Autodesk Inventor part; units mm, degrees
ref_plane "YZ Plane" through (0, 0, 0) normal (1, 0, 0) x (0, 1, 0)
ref_plane "XZ Plane" through (0, 0, 0) normal (0, 1, 0) x (-1, 0, 0)
ref_plane "XY Plane" through (0, 0, 0) normal (0, 0, 1) x (1, 0, 0)
sketch "Sketch1" plane through (0, 0, 0) normal (0, 0, 1) x (1, 0, 0)
  line L0 (-2.6473, 22.1) -> (2.6473, 22.1)
  line L1 (2.6473, 22.1) -> (2.6473, 12)
  line L2 (2.6473, 12) -> (4.1473, 12)
  line L3 (4.1473, 12) -> (4.1473, 4.1473)
  line L4 (0, 22.1) -> (0, 0) construction
  line L5 (-2.6473, 22.1) -> (-2.6473, 12)
  line L6 (-2.6473, 12) -> (-4.1473, 12)
  line L7 (-1.25, 18.6) -> (1.25, 18.6)
  line L8 (1.25, 18.6) -> (1.25, 17.5)
  line L9 (1.25, 17.5) -> (-1.25, 17.5)
  line L10 (-1.25, 17.5) -> (-1.25, 18.6)
  line L11 (-9.6473, -24) -> (16.1473, -24)
  line L12 (26.1473, -9) -> (16.1473, -9)
  line L13 (16.1473, -9) -> (16.1473, -24)
  line L14 (3.0473, 2.1473) -> (4.1473, 2.1473)
  line L15 (4.1473, 2.1473) -> (4.1473, -0.3527)
  line L16 (4.1473, -0.3527) -> (3.0473, -0.3527)
  line L17 (3.0473, -0.3527) -> (3.0473, 2.1473)
  line L18 (-4.1473, 12) -> (-30.8527, 12) construction
  line L19 (-27.6, 2.6473) -> (-27.6, -2.6473)
  line L20 (-27.6, -2.6473) -> (-17.5, -2.6473)
  line L21 (-17.5, -2.6473) -> (-17.5, -4.1473)
  line L22 (-17.5, -4.1473) -> (-9.6473, -4.1473)
  line L23 (-9.6473, -4.1473) -> (-9.6473, -24)
  line L24 (-27.6, 2.6473) -> (-17.5, 2.6473)
  line L25 (-17.5, 2.6473) -> (-17.5, 4.1473)
  line L26 (-24.1, 1.25) -> (-24.1, -1.25)
  line L27 (-24.1, -1.25) -> (-23, -1.25)
  line L28 (-23, -1.25) -> (-23, 1.25)
  line L29 (-23, 1.25) -> (-24.1, 1.25)
  line L30 (-17.5, 12) -> (-17.5, -24) construction
  line L31 (-4.1473, 12) -> (-4.1473, 4.1473)
  line L32 (-9.6473, 4.1473) -> (-17.5, 4.1473)
  line L33 (-4.1473, 4.1473) -> (-9.6473, 4.1473)
  line L34 (26.1473, 4.1473) -> (26.1473, -9)
  line L35 (26.1473, -2.4263) -> (4.1473, -2.4263) construction
  line L36 (3.0473, -7) -> (4.1473, -7)
  line L37 (4.1473, -7) -> (4.1473, -4.5)
  line L38 (4.1473, -4.5) -> (3.0473, -4.5)
  line L39 (3.0473, -4.5) -> (3.0473, -7)
  line L40 (4.1473, 4.1473) -> (26.1473, 4.1473)
  point P0 (0, 17.5)
  point P1 (3.0473, 0.8973)
  point P2 (4.1473, 0.8973)
  point P3 (-24.1, 0)
  point P4 (-27.6, 0)
  dimension "d4" = 1.5
  dimension "d26" = 10.1
  dimension "d27" = 5.2946
  dimension "d31" = 2.5
  dimension "d32" = 1.1
  dimension "d35" = 5.5
  dimension "d41" = 1.1
  dimension "d42" = 2.5
  dimension "d72" = 17.5
  dimension "BearingHolderHeight" = 24.5263
  dimension "d99" = 5.5
  dimension "d103" = 12
  dimension "d104" = 10
  dimension "d105" = 13.1473
  dimension "d106" = 2
  dimension "d108" = 15
  dimension "d124" = 12
  dimension "d125" = 7.8527
extrude "Extrusion2" add sketch "Sketch1" along normal blind 6.39
equation "\"BearingDiameter\" = 24"
equation "\"WoodThickness\" = 6.39"
equation "\"BearingWidth\" = 7"
equation "\"BearingShaftDiameter\" = 8"
equation "\"ZipTieWidth\" = 2.5"
equation "\"ZipTieThickness\" = 1.1"
equation "\"ZipTieClearance\" = 1"
equation "\"ZipTieDistance\" = 10"
equation "\"BearingSiliconeWidth\" = 14"
properties part number "BearingStand_V2" material "Wood (Birch)"
Check sheet for the modelled part. Datum: model origin and axes. Units: mm. A direction names the side the tool comes from. Give positions to 0.01 mm unless a question says otherwise; leave off trailing zeros. Order: outer loops, then holes, each group sorted by start corner. A loop starts at its lowest first (then second) coordinate and runs counter-clockwise, first axis right, second up. Notation, with made-up numbers: M 36.25,-13.75 L 89.25,-13.75 A17 cw 89.25,15.25 Z; hole C -19,3 d10. An arc over 180 degrees is marked long. Answer in a Markdown table with one row per item.
1) Cross-section at B-B, the plane x = 19.5. Enter the section's corners in (y, z), plus the area to 3 significant figures.
Filled sheet:
| item | result |
|---|---|
| outline | M -9,0 L 4.15,0 L 4.15,6.39 L -9,6.39 Z |
| area | 84.0 mm2 |
2) Access from +Z, -Z, +X, -X, +Y, -Y to the whole of each face (thin tool, end or side, straight path). Record for faces 5 (the flat face through (15, 4.147, 3)), 6 (the flat face through (21, -9, 3)), 7 (the flat face through (-23.6, -1.25, 3.2)).
Filled sheet:
| item | result |
|---|---|
| face 5 | +Z, -Z, +X, +Y |
| face 6 | +Z, -Z, +X, -Y |
| face 7 | +Z, -Z |
3) Gauge pin test, flat ends, axial feed: P1, Ø0.9, axis at y = 18.5, z = 2, coming from the -X side; P2, Ø1.9, axis at x = 20.5, z = 2, coming from the +Y side; P3, Ø1.9, axis at y = 8, z = 2.5, coming from the +X side. Record the tip position at first contact, or that the pin passes through.
Filled sheet:
| item | result |
|---|---|
| P1 | stops at x = -2.65 |
| P2 | stops at y = 4.15 |
| P3 | stops at x = 4.15 |
4) Cross-section at A-A, the plane z = 2. Count the separate pieces of the cut face and the enclosed holes in it, plus the area to 3 significant figures.
Filled sheet:
| item | result |
|---|---|
| separate pieces | 1 |
| enclosed holes | 4 |
| area | 1,080 mm2 |
5) Cross-section at C-C, the plane y = -3.5. Enter the section's corners in (x, z), plus the area to 3 significant figures.
Filled sheet:
| item | result |
|---|---|
| outline | M -17.5,0 L 26.15,0 L 26.15,6.39 L -17.5,6.39 Z |
| area | 279 mm2 |
6) Release check for a two-part mould opening along X. For faces 1 (the flat face through (16.147, -16, 3)), 2 (the flat face through (-1.25, 18, 3)), 3 (the flat face through (-11, 4.147, 3)), 4 (the flat face through (3.047, -6, 3)) record: +X half, -X half, draft (parallel to the pull), parting line (faces both ways), or undercut.
Filled sheet:
| item | result |
|---|---|
| face 1 | +X half |
| face 2 | undercut |
| face 3 | draft |
| face 4 | undercut |
7) Thickness scan on L1, parallel to X at y = 0, z = 2; L2, parallel to X at y = -5, z = 5.5; L3, parallel to Y at x = -5.5, z = 0.5. Record the ranges inside material, lowest first. Write a range as [from, to].
Filled sheet:
| item | result |
|---|---|
| L1 | x = [-27.6, -24.1], [-23, 3.05], [4.15, 26.15] |
| L2 | x = [-9.65, 3.05], [4.15, 26.15] |
| L3 | y = [-24, 4.15] |
